```python
from build123d import *

# Parameters (mm, degrees)
F1_DEPTH = 12.7
F2_W     = 184.15
F2_H     = 116.4964555132
F3_DEPTH = 19.05
F4_DEPTH = 25.4
F5_W     = 38.1
F5_H     = 12.7
F6_DEPTH = 12.7


with BuildPart() as f1:
    # F0 (on Top) → F1 (new body)
    with BuildSketch(Plane.XY):
        with BuildLine():
            Line((98.2942968156, 10.920933083), (110.9942968156, 10.920933083))
            Line((110.9942968156, 10.920933083), (110.9942968156, -14.479066917))
            Line((110.9942968156, -14.479066917), (149.0942968156, -14.479066917))
            Line((149.0942968156, -14.479066917), (149.0942968156, 23.620933083))
            Line((149.0942968156, 23.620933083), (257.0442968156, 23.620933083))
            Line((257.0442968156, 23.620933083), (257.0442968156, 58.545933083))
            ThreePointArc((257.0442968156, 58.545933083), (177.2761177053, 76.6173885961), (98.2942968156, 55.370933083))
            Line((98.2942968156, 55.370933083), (98.2942968156, 10.920933083))
        make_face()
    extrude(amount=F1_DEPTH)

    # F2 (on face) → F3 (join)
    with BuildSketch(Plane(origin=(0, 0, 0), x_dir=(1, 0, 0), z_dir=(0, 0, -1))):
        with Locations((177.6692968156, -31.0691608395)):
            Rectangle(F2_W, F2_H)
    extrude(amount=F3_DEPTH)

    # F4 (cut): a face of the model
    f4_faces = [f1.faces().sort_by_distance(p)[0] for p in [
        (169.3940346963, 39.8760079107, 12.7),
    ]]
    extrude(f4_faces, amount=-F4_DEPTH, mode=Mode.SUBTRACT)

    # F5 (on face) → F6 (cut)
    with BuildSketch(Plane.XY):
        with Locations((130.0442968156, -20.829066917)):
            Rectangle(F5_W, F5_H)
    extrude(amount=-F6_DEPTH, mode=Mode.SUBTRACT)


solid = f1.part
```
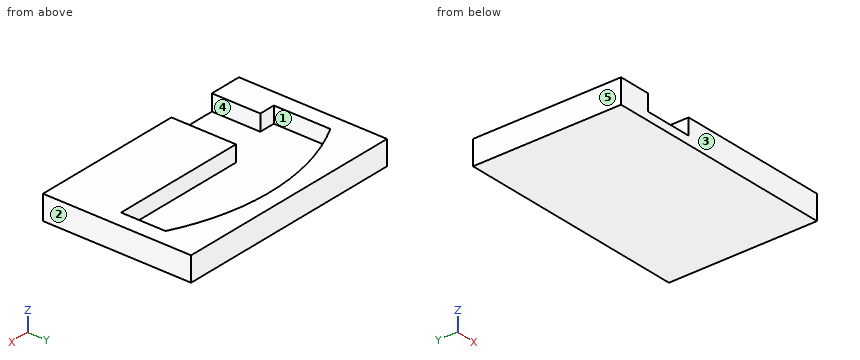
Design review of the part built by this model. Coordinates are the model's own, in mm. Face numbers are marked on the shaded views. A direction names the side the tool comes from. Coordinates: 2 decimals unless noted, no trailing zeros. Write each loop counter-clockwise with the first axis right and the second up, starting at its lowest first coordinate (ties: lowest second). Pieces come first, ordered by that corner, then holes. Notation, with made-up numbers: M -33,63 L 9,63 A23 cw 9,100 Z; hole C 81,28.5 d7. An arc over 180 degrees is marked long. Answer as a JSON object with one key per item and string values.
Item 1: Add section A-A, the plane z = -8.75. Give the boundary of the cut face in (x, y), and give its area (3 significant figures).
Outcome:
{"outline": "M 85.59,-27.18 L 110.99,-27.18 L 110.99,10.92 L 98.29,10.92 L 98.29,55.37 A170.11 cw 257.04,58.55 L 257.04,23.62 L 149.09,23.62 L 149.09,-27.18 L 269.74,-27.18 L 269.74,89.32 L 85.59,89.32 Z", "area": "12,000 mm²"}
Item 2: Draft analysis for pull direction X (two halves, no side actions). For the marked faces 3, 4 and 5, state which applies: pulls with the +X half, pulls with the -X half, needs draft (parallel to the pull), parting line crosses it, or undercut.
Outcome:
{"face 3": "needs draft", "face 4": "undercut", "face 5": "pulls with the -X half"}
Item 3: Insertion check: pin 1 Ø3 at (x, z) = (121.5, -8.5) entering from -Y; pin 2 Ø3 at (x, y) = (138.5, 3.5) entering from +Z; pin 3 Ø10 at (x, y) = (173.5, 10.5) entering from +Z. Each pin has a flat end and moves straight along its axis. Give the tip position at first contact, or say it passes through.
Outcome:
{"pin 1": "y = 65.46", "pin 2": "z = -12.7", "pin 3": "z = 0"}
Item 4: Add section B-B, the plane y = 48. Give the boundary of the cut face in (x, z), and give its area (3 significant figures).
Outcome:
{"outline": "M 85.59,-19.05 L 269.74,-19.05 L 269.74,0 L 257.04,0 L 257.04,-12.7 L 98.29,-12.7 L 98.29,0 L 85.59,0 Z", "area": "1,490 mm²"}
Item 5: Machinability: for the marked faces 1 and 2, which of the approach directions +Z, -Z, +X, -X, +Y, -Y give a long, thin tool a straight path to every point of the face, cutting with its end or side? Answer none if there is none.
Outcome:
{"face 1": "+Z", "face 2": "+Z, -Z, +X, +Y, -Y"}
Item 6: Add section C-C, the plane x = 199. Give the boundary of the cut face in (y, z), and give its area (3 significant figures).
Outcome:
{"outline": "M -27.18,-19.05 L 89.32,-19.05 L 89.32,0 L 75.66,0 L 75.66,-12.7 L 23.62,-12.7 L 23.62,0 L -27.18,0 Z", "area": "1,560 mm²"}
Item 7: Add section D-D, the plane x = 119.5. Give the boundary of the cut face in (y, z).
Outcome:
{"outline": "M -27.18,-19.05 L 89.32,-19.05 L 89.32,0 L 65.27,0 L 65.27,-12.7 L -27.18,-12.7 Z"}
Item 8: Wall thickness on probe 1 along X at (y, z) = (9.5, -1.75); probe 2 along X at (y, z) = (38.5, -2.25); probe 3 along Z at (x, y) = (134.5, -13): over which ranges is each line inside the solid? List them lowest first.
Outcome:
{"probe 1": "85.59 to 110.99, 149.09 to 269.74", "probe 2": "85.59 to 98.29, 257.04 to 269.74", "probe 3": "-19.05 to -12.7"}
